Read the model definition and answer for the solid it produces. Units are mm, in the model's axes. A direction names the side the tool comes from. Round coordinates to 2 decimals unless told otherwise and drop trailing zeros. Write each loop counter-clockwise with the first axis right and the second up, starting at its lowest first coordinate (ties: lowest second). Pieces come first, ordered by that corner, then holes. Notation, with made-up numbers: (80.25, -6.5) -> (129.25, -6.5) arc R7 cw to (129.25, 2.5) -> close; hole circle Ø2 at (51, -9.75). An arc over 180 degrees is marked (long way). Return JSON: item names as keys, results as strings.
from build123d import *

# Parameters (mm, degrees)
BOSS_EXTRUDE1_DEPTH = 22.5
SKETCH2_OUTSIDE_W   = 294.908
SKETCH2_OUTSIDE_H   = 310.996
SKETCH2_OUTSIDE_R   = 52
CUT_EXTRUDE1_DEPTH  = 45
CUT_EXTRUDE1_DRAFT  = -60
SKETCH3_OUTSIDE_W   = 294.908
SKETCH3_OUTSIDE_H   = 310.996
SKETCH3_OUTSIDE_R   = 52
CUT_EXTRUDE2_DEPTH  = 45
CUT_EXTRUDE2_DRAFT  = -60
SKETCH4_R           = 25
BOSS_EXTRUDE2_DEPTH = 400
FILLET1_R           = 4


with BuildPart() as part:
    # Sketch1 → Boss-Extrude1 (new, symmetric)
    with BuildSketch(Plane.XY):
        Polygon((52, 30.022213998), (0, 60.044427996), (-52, 30.022213998), (-52, -30.022213998), (0, -60.044427996), (52, -30.022213998), align=None)
    extrude(amount=BOSS_EXTRUDE1_DEPTH, both=True)


with BuildPart() as cut_extrude1_tool:
    # Sketch2 outside → Cut-Extrude1 (with draft: the straight prism first)
    with BuildSketch(Plane.XY.offset(22.5)):
        Rectangle(SKETCH2_OUTSIDE_W, SKETCH2_OUTSIDE_H)
        Circle(SKETCH2_OUTSIDE_R, mode=Mode.SUBTRACT)
    extrude(amount=-CUT_EXTRUDE1_DEPTH)
    # Cut-Extrude1: the draft: its side faces are tilted about the plane it starts from
    cut_extrude1_sides = [cut_extrude1_tool.faces().sort_by_distance(p)[0] for p in [
        (0, -155.498, 0),
        (147.454, 0, 0),
        (0, 155.498, 0),
        (-147.454, 0, 0),
        (-52, 0, 0),
    ]]
    draft(cut_extrude1_sides, Plane.XY.offset(22.5), CUT_EXTRUDE1_DRAFT)


with BuildPart() as part_1:
    add(part.part)

    # Cut-Extrude1: cut by cut_extrude1_tool
    add(cut_extrude1_tool.part, mode=Mode.SUBTRACT)


with BuildPart() as cut_extrude2_tool:
    # Sketch3 outside → Cut-Extrude2 (with draft: the straight prism first)
    with BuildSketch(Plane(origin=(0, 0, -22.5), x_dir=(-1, 0, 0), z_dir=(0, 0, -1))):
        Rectangle(SKETCH3_OUTSIDE_W, SKETCH3_OUTSIDE_H)
        Circle(SKETCH3_OUTSIDE_R, mode=Mode.SUBTRACT)
    extrude(amount=-CUT_EXTRUDE2_DEPTH)
    # Cut-Extrude2: the draft: its side faces are tilted about the plane it starts from
    cut_extrude2_sides = [cut_extrude2_tool.faces().sort_by_distance(p)[0] for p in [
        (0, -155.498, 0),
        (-147.454, 0, 0),
        (0, 155.498, 0),
        (147.454, 0, 0),
        (52, 0, 0),
    ]]
    draft(cut_extrude2_sides, Plane(origin=(0, 0, -22.5), x_dir=(-1, 0, 0), z_dir=(0, 0, -1)), CUT_EXTRUDE2_DRAFT)


with BuildPart() as part_2:
    add(part_1.part)

    # Cut-Extrude2: cut by cut_extrude2_tool
    add(cut_extrude2_tool.part, mode=Mode.SUBTRACT)

    # Sketch4 → Boss-Extrude2 (add)
    with BuildSketch(Plane(origin=(0, 0, -22.5), x_dir=(-1, 0, 0), z_dir=(0, 0, -1))):
        with Locations(Location((0, 0, 0), (0, 0, 180))):
            Circle(SKETCH4_R)
    extrude(amount=BOSS_EXTRUDE2_DEPTH)

    # Fillet1
    fillet1_edges = [part_2.edges().sort_by_distance(p)[0] for p in [
        (-25, 0, -422.5),
    ]]
    fillet(fillet1_edges, radius=FILLET1_R)


solid = part_2.part
Item 1: Section A-A (z = -182) is taken. Give the vertices of the cut face in (x, y), then the cut area to 3 significant figures.
Worked answers:
{"outline": "circle Ø50 at (0, 0)", "area": "1,960 mm2"}
Item 2: Flat-ended cylindrical pins translate along their axes: pin 1 (2 mm diameter, centred on x = 27.5, y = 15.5, fed in from -Z); pin 2 (5 mm diameter, centred on y = -24.5, z = -186.5, fed in from -X); pin 3 (1.5 mm diameter, centred on x = 21.5, z = -260, fed in from -Y). Find the tip coordinate at first contact, or state that the pin passes through.
Worked answers:
{"pin 1": "stops at z = -22.5", "pin 2": "stops at x = -11.87", "pin 3": "stops at y = -13.94"}
Item 3: Straight lines are drawn through the part: L1, parallel to Y at x = 17.5, z = -193; L2, parallel to Z at x = -19, y = 40; L3, parallel to Z at x = 23.5, y = 6.5. For each, find the intervals that lie inside material, in ascending order. Write a range as [from, to].
Worked answers:
{"L1": "y = [-17.85, 17.85]", "L2": "z = [-22.5, 22.5]", "L3": "z = [-420.64, 22.5]"}
Item 4: A tool of negligible diameter and unlimited length cuts with its end or side. For faces 1 (the conical face through (46.76, -26.845, -21.393)), 2 (the flat face through (22.4, 12.3, -22.5)), from which of +Z, -Z, +X, -X, +Y, -Y can it reach the whole face along a straight path? Write none if from no direction.
Worked answers:
{"face 1": "-Z, +X, -Y", "face 2": "-Z"}
